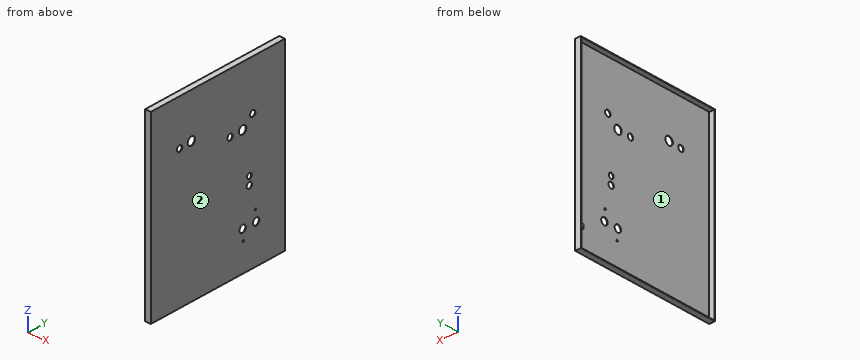
Autodesk Inventor part; units mm, degrees
ref_plane "YZ Plane" through (0, 0, 0) normal (1, 0, 0) x (0, 1, 0)
ref_plane "XZ Plane" through (0, 0, 0) normal (0, 1, 0) x (-1, 0, 0)
ref_plane "XY Plane" through (0, 0, 0) normal (0, 0, 1) x (1, 0, 0)
sketch "Sketch1" plane through (0, 0, 0) normal (0, 0, 1) x (1, 0, 0)
  circle A0 centre (-73.5453, -435.8173) radius 2.15
  circle A1 centre (-73.5453, -435.8173) radius 2.8
  line L0 (-76.3453, -435.8173) -> (-70.7453, -435.8173)
  line L1 (-70.7453, -435.8173) -> (-70.7453, -430.8173)
  line L2 (-70.7453, -430.8173) -> (-76.3453, -430.8173)
  line L3 (-76.3453, -430.8173) -> (-76.3453, -435.8173)
  point P0 (0, 0)
  dimension "d1" = 5.6
  dimension "d2" = 5
extrude "Extrusion1" add sketch "Sketch1" along normal blind 10 contours L0 A1 A0 | A0 L0 A1 | A1 L3 L2 L1
sketch "Sketch2" plane through (-76.3453, -430.8173, 0) normal (0, 1, 0) x (1, 0, 0)
  line L0 (0, 49.3) -> (14, 49.3)
  line L1 (14, 49.3) -> (14, -439.7)
  line L2 (14, -439.7) -> (0, -439.7)
  line L3 (0, -439.7) -> (0, 49.3)
  line L4 (-11.8992, -390) -> (-11.8992, -380)
  line L5 (-11.8992, -380) -> (0.8131, -380)
  line L6 (0.8131, -380) -> (0.8131, -390)
  line L7 (0.8131, -390) -> (-11.8992, -390)
  line L8 (-11.8992, 0) -> (-11.8992, 10)
  line L9 (-11.8992, 10) -> (0.8131, 10)
  line L10 (0.8131, 10) -> (0.8131, 0)
  line L11 (0.8131, 0) -> (-11.8992, 0)
  line L12 (1.6631, -425.4) -> (1.6631, 35)
  line L13 (1.6631, 35) -> (308.0179, 35)
  line L14 (308.0179, 35) -> (308.0179, -425.4)
  line L15 (308.0179, -425.4) -> (1.6631, -425.4)
  line L16 (322.7236, -442.7) -> (322.7236, 52.3)
  line L17 (322.7236, 52.3) -> (-13.0426, 52.3)
  line L18 (-13.0426, 52.3) -> (-13.0426, -442.7)
  line L19 (-13.0426, -442.7) -> (322.7236, -442.7)
  point P0 (76.3453, 0)
  point P1 (0, -10)
  dimension "d5" = 14
  dimension "d6" = 489
  dimension "d7" = 3
  dimension "d8" = 3
extrude "Extrusion2" add sketch "Sketch2" along normal blind 1.6 contours L0 L1 L13 L12 L15 L2 L3 L7 L6 L5 L11 L10 L9 | L9 L10 L11 L3 | L1 L15 L12 L13 | L5 L6 L7 L3
sketch "Sketch3" plane through (-62.3453, -430.8173, 439.7) normal (1, 0, 0) x (0, 0, -1)
  line L0 (489, 0) -> (489, 1.6)
  line L1 (489, 1.6) -> (0, 1.6)
  line L2 (0, 1.6) -> (0, -394.4)
  line L3 (0, -394.4) -> (489, -394.4)
  line L4 (489, -394.4) -> (489, 1.6)
  point P0 (439.7, 430.8173)
  point P1 (489, 0)
  dimension "d11" = 396
extrude "Extrusion3" add sketch "Sketch3" along normal blind 1.6
sketch "Sketch4" plane through (-62.3453, -430.8173, 439.7) normal (-1, 0, 0) x (0, 0, 1)
  line L0 (0, 0) -> (-1.6, 0)
  line L1 (-1.6, 0) -> (-1.6, -394.4)
  line L2 (-1.6, -394.4) -> (0, -394.4)
  line L3 (0, -394.4) -> (0, 0)
  line L4 (-1.6, -392.8) -> (-489, -392.8)
  line L5 (-489, -392.8) -> (-489, -394.4)
  line L6 (-489, -394.4) -> (-1.6, -394.4)
  line L7 (-1.6, -394.4) -> (-1.6, -392.8)
  line L8 (-487.4, 0) -> (-489, 0)
  line L9 (-489, 0) -> (-489, -394.4)
  line L10 (-489, -394.4) -> (-487.4, -394.4)
  line L11 (-487.4, -394.4) -> (-487.4, 0)
  point P0 (-439.7, 430.8173)
  point P1 (0, -394.4)
  point P2 (-489, -394.4)
  point P3 (0, 0)
  point P4 (-487.4, -392.8)
  point P5 (-489, -392.8)
  point P6 (-1.6, -394.4)
  dimension "d14" = 1.6
  dimension "d15" = 1.6
  dimension "d16" = 1.6
extrude "Extrusion4" add sketch "Sketch4" along normal up to surface (14 mm away)
sketch "Sketch5" plane through (-60.7453, -430.8173, 439.7) normal (1, 0, 0) x (0, 0, -1)
  circle A0 centre (118.4923, -274.4067) radius 11
  circle A1 centre (120.9923, -309.4067) radius 8
  circle A2 centre (158.3816, -160.3944) radius 8
  circle A3 centre (157.195, -123.3944) radius 11
  circle A4 centre (132.195, -93.3944) radius 8
  circle A5 centre (271.7988, -103.395) radius 7.05
  circle A6 centre (293.6378, -103.395) radius 8
  circle A7 centre (414.1683, -121.0429) radius 2.3
  circle A8 centre (414.1683, -121.0429) radius 2.3
  circle A9 centre (385.3683, -123.0429) radius 9.5
  circle A10 centre (356.5683, -85.3929) radius 2.3
  circle A11 centre (385.3683, -83.3929) radius 9.5
  point P0 (439.7, 430.8173)
extrude "Extrusion5" cut sketch "Sketch5" along normal mid plane 100
properties part number "door"
The model under review builds one solid part; all positions refer to its coordinate system, in mm. Face numbers are marked on the shaded views. Round coordinates to 2 decimals unless told otherwise and drop trailing zeros. Loops run counter-clockwise (first coordinate to the right, second up) from the corner with the lowest first, then second, coordinate; pieces in that order, holes last.
Item 1: Clearance check with flat-ended pins moving along their axes: pin 1 Ø5.5 at (y, z) = (-516.21, 83.13) entering from +X; pin 2 Ø16 at (y, z) = (-534.21, 167.9) entering from -X. State where each tip first meets the part, or that it passes through.
Determined:
pin 1: stops at x = -60.75
pin 2: stops at x = -62.35
Item 2: Take a section at A-A (z = 355.5). Write out the cut boundary in (x, y).
Determined:
outline: (-76.35, -825.22) - (-60.75, -825.22) - (-60.75, -429.22) - (-76.35, -429.22) - (-76.35, -430.82) - (-62.35, -430.82) - (-62.35, -823.62) - (-76.35, -823.62) - close
Item 3: For line 1 (Y direction, x = -65, z = 151.5); line 2 (Z direction, x = -68.5, y = -495); line 3 (X direction, y = -557.5, z = 177.5), list the stretches that pass through material, from the lowest coordinate up.
Determined:
line 1: y = -825.22 to -823.62, -430.82 to -429.22
line 2: z = -49.3 to -47.7, 438.1 to 439.7
line 3: x = -62.35 to -60.75
Item 4: Mouldability with a two-part tool opening along Y and no side actions: class the marked faces 1 and 2 as released by +Y, released by -Y, zero draft, split by the parting line, or undercut.
Determined:
face 1: undercut
face 2: zero draft
Item 5: Take a section at B-B (y = -607). Write out the cut boundary in (x, z), then the cut area to 3 significant figures.
Determined:
outline: (-76.35, -49.3) - (-60.75, -49.3) - (-60.75, 439.7) - (-76.35, 439.7) - (-76.35, 438.1) - (-62.35, 438.1) - (-62.35, -47.7) - (-76.35, -47.7) - close
area: 827 mm2
